```python
from build123d import *

# Parameters (mm, degrees)
BOSS_EXTRUDE1_DEPTH = 10


with BuildPart() as part:
    # Sketch1 → Boss-Extrude1 (new body)
    with BuildSketch(Plane(origin=(0, 0, 0), x_dir=(1, 0, 0), z_dir=(0, 1, 0))):
        with BuildLine():
            Line((150, 0), (150, 40))
            Line((150, 40), (170, 40))
            ThreePointArc((170, 40), (190, 20), (170, 0))
            Line((170, 0), (150, 0))
        make_face()
        with BuildLine():
            Line((170, 32), (158, 32))
            Line((158, 32), (158, 8))
            Line((158, 8), (170, 8))
            ThreePointArc((170, 8), (182, 20), (170, 32))
        make_face(mode=Mode.SUBTRACT)
    extrude(amount=BOSS_EXTRUDE1_DEPTH)


solid = part.part
```
Input: part model. Units: mm. Frame: model coordinates. A direction names the side the tool comes from. Round coordinates to 2 decimals unless told otherwise and drop trailing zeros. Write each loop counter-clockwise with the first axis right and the second up, starting at its lowest first coordinate (ties: lowest second). Pieces come first, ordered by that corner, then holes. Notation, with made-up numbers: M -22.5,75.25 L 3.5,75.25 A19 cw 3.5,99.25 Z; hole C 22,25 d4. An arc over 180 degrees is marked long. Write each question's results on one line, items separated by ' | '.
Q1. Section query D-D (x = 186). Return loops of the section in (y, z).
Results:
outline: M 0,-32 L 10,-32 L 10,-8 L 0,-8 Z
Q2. Draft query along X for faces 3 (the face through (190, 5, -20)), 4 (the face through (182, 5, -20)), 5 (the face through (164, 5, -8)), 6 (the face through (157, 10, -20)). Return one class per face: released by +X, released by -X, zero draft, split by the parting line, or undercut.
Results:
face 3: released by +X | face 4: undercut | face 5: undercut | face 6: zero draft
Q3. Section query B-B (y = 0.5). Return loops of the section in (x, z), and give its area (3 significant figures).
Results:
outline: M 150,-40 L 170,-40 A20 ccw 170,0 L 150,0 Z; hole M 158,-32 L 170,-32 A12 ccw 170,-8 L 158,-8 Z | area: 914 mm^2
Q4. Section query C-C (x = 180.5). Return loops of the section in (y, z), and give its area (3 significant figures).
Results:
outline: M 0,-37.02 L 10,-37.02 L 10,-25.81 L 0,-25.81 Z; M 0,-14.19 L 10,-14.19 L 10,-2.98 L 0,-2.98 Z | area: 224 mm^2
Q5. Section query A-A (z = -20). Return loops of the section in (x, y).
Results:
outline: M 150,0 L 158,0 L 158,10 L 150,10 Z; M 182,0 L 190,0 L 190,10 L 182,10 Z
Q6. Pin query (flat end, axial travel): P1, Ø5, axis at x = 164.5, y = 5.5, coming from the +Z side; P2, Ø3, axis at y = 7, z = -23, coming from the +X side; P3, Ø2, axis at y = 2, z = -21, coming from the +X side. Return the tip coordinate at first contact, or that it passes through.
Results:
P1: stops at z = 0 | P2: stops at x = 189.94 | P3: stops at x = 190
Q7. Access query for faces 1 (the face through (160, 5, 0)), 2 (the face through (164, 5, -32)). Directions: +Z, -Z, +X, -X, +Y, -Y. A direction counts if a zero-diameter tool reaches every point of the face in a straight line with its end or side. Return the directions, or none.
Results:
face 1: +Z, +X, -X, +Y, -Y | face 2: +Y, -Y
Q8. Line query: line 1 along Z through (x, y) = (162, 5); line 2 along X through (y, z) = (5.5, -13) (3 decimals); line 3 along X through (y, z) = (4.75, -9). Output: solid intervals per line, ascending.
Results:
line 1: z = -40 to -32, -8 to 0 | line 2: x = 150 to 158, 179.747 to 188.735 | line 3: x = 150 to 158, 174.8 to 186.7
